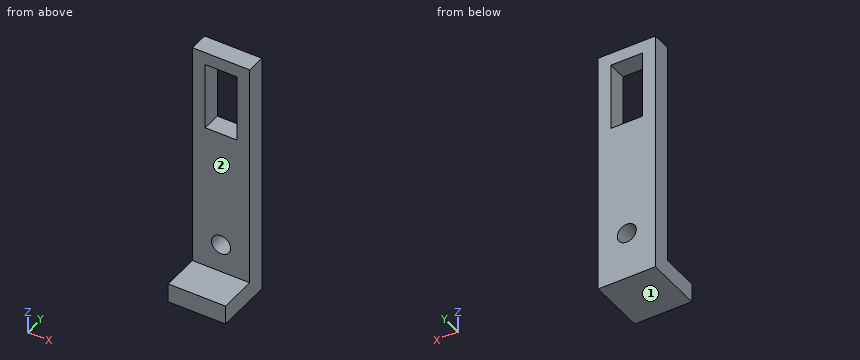
```python
from build123d import *

# Parameters (mm, degrees)
SKETCH1_W           = 9
SKETCH1_H           = 35.7
SKETCH1_R           = 1.5
BOSS_EXTRUDE1_DEPTH = 3
SKETCH2_W           = 9
SKETCH2_H           = 3
BOSS_EXTRUDE2_DEPTH = 9


with BuildPart() as part:
    # Sketch1 → Boss-Extrude1 (new body)
    with BuildSketch(Plane(origin=(0, 0, 0), x_dir=(1, 0, 0), z_dir=(0, 1, 0))):
        with Locations((-4.5, -17.85)):
            Rectangle(SKETCH1_W, SKETCH1_H)
        with Locations(Location((-4.5, -4.5, 0), (0, 0, 270))):
            Circle(SKETCH1_R, mode=Mode.SUBTRACT)
        Polygon((-7, -32.7), (-7, -33.7), (-2, -33.7), (-2, -32.7), (-2, -23.1), (-7, -23.1), align=None, mode=Mode.SUBTRACT)
    extrude(amount=BOSS_EXTRUDE1_DEPTH)

    # Sketch2 → Boss-Extrude2 (add)
    with BuildSketch(Plane(origin=(0, 3, 0), x_dir=(1, 0, 0), z_dir=(0, 1, 0))):
        with Locations((-4.5, 1.5)):
            Rectangle(SKETCH2_W, SKETCH2_H)
    extrude(amount=-BOSS_EXTRUDE2_DEPTH)


solid = part.part
```
Verification items for the finished model (mm, model axes). Face numbers are marked on the shaded views. A direction names the side the tool comes from. Coordinates: 2 decimals unless noted, no trailing zeros. Loops run counter-clockwise (first coordinate to the right, second up) from the corner with the lowest first, then second, coordinate; pieces in that order, holes last. Notation, with made-up numbers: (45, 72.5) - (58, 72.5) arc R19 cw to (58, 80.5) - close; hole circle Ø7 at (79, 13.25). An arc over 180 degrees is marked (long way). Return JSON: item names as keys, results as strings.
1. Thickness scan on L1, parallel to X at y = 2.2, z = 4.5; L2, parallel to Z at x = -5, y = 1.5; L3, parallel to Z at x = -3.5, y = 0.5. Record the ranges inside material, lowest first.
Established:
{"L1": "x = -9 to -6, -3 to 0", "L2": "z = -3 to 3.09, 5.91 to 23.1, 33.7 to 35.7", "L3": "z = -3 to 3.38, 5.62 to 23.1, 33.7 to 35.7"}
2. Go/stop test with flat-tipped pins: pin 1 (3 mm diameter, centred on x = -5.5, y = -3, fed in from +Z); pin 2 (3.5 mm diameter, centred on y = 1, z = 26, fed in from +X); pin 3 (1.5 mm diameter, centred on x = -7, z = 3, fed in from -Y). Record where each tip stops, or that it passes through.
Established:
{"pin 1": "stops at z = 0", "pin 2": "stops at x = 0", "pin 3": "stops at y = 0"}
3. Tool access check on the marked faces 1 and 2. Record the directions out of +Z, -Z, +X, -X, +Y, -Y that give a thin tool (end or side, any length) a straight path to the whole face; none if there is none.
Established:
{"face 1": "-Z, +X, -X, +Y, -Y", "face 2": "+Z, +X, -X, -Y"}
4. Section check B-B, the plane x = -4.5. Record the boundary of the cut face in (y, z), then the cut area to 3 significant figures.
Established:
{"outline": "(-6, -3) - (3, -3) - (3, 3) - (0, 3) - (0, 0) - (-6, 0) - close; (0, 6) - (3, 6) - (3, 23.1) - (0, 23.1) - close; (0, 33.7) - (3, 33.7) - (3, 35.7) - (0, 35.7) - close", "area": "93.3 mm2"}
5. Section check D-D, the plane y = -5. Record the boundary of the cut face in (x, z), then the cut area to 3 significant figures.
Established:
{"outline": "(-9, -3) - (0, -3) - (0, 0) - (-9, 0) - close", "area": "27.0 mm2"}
6. Section check A-A, the plane z = 4.5. Record the boundary of the cut face in (x, y), then the cut area to 3 significant figures.
Established:
{"outline": "(-9, 0) - (-6, 0) - (-6, 3) - (-9, 3) - close; (-3, 0) - (0, 0) - (0, 3) - (-3, 3) - close", "area": "18.0 mm2"}
7. Section check C-C, the plane z = 27. Record the boundary of the cut face in (x, y).
Established:
{"outline": "(-9, 0) - (-7, 0) - (-7, 3) - (-9, 3) - close; (-2, 0) - (0, 0) - (0, 3) - (-2, 3) - close"}
